Geometry check sheet. Reference: the model listing, model coordinates, mm. A direction names the side the tool comes from. Round coordinates to 2 decimals unless told otherwise and drop trailing zeros. Order: outer loops, then holes, each group sorted by start corner. A loop starts at its lowest first (then second) coordinate and runs counter-clockwise, first axis right, second up. Notation, with made-up numbers: (-1, -5.5) -> (29, -5.5) arc R8 cw to (29, -0.5) -> close; hole circle Ø7 at (-19, -28.75). An arc over 180 degrees is marked (long way). Answer as a JSON object with one key per item and string values. Group by question number.
Autodesk Inventor part; units mm, degrees
ref_plane "工作平面1" through (0, 3.5, 0) normal (0, 1, 0) x (-1, 0, 0)
ref_plane "YZ Plane" through (0, 0, 0) normal (1, 0, 0) x (0, 1, 0)
ref_plane "XY Plane" through (0, 0, 0) normal (0, 0, 1) x (1, 0, 0)
sketch "草圖1" plane through (0, 0, 0) normal (0, 1, 0) x (-1, 0, 0)
  circle A0 centre (0, 0) radius 1.75
  arc A1 (5, 0) -> (-5, 0) centre (0, 0) ccw
  circle A2 centre (0, -50) radius 1.75
  arc A3 (-5, -50) -> (5, -50) centre (0, -50) ccw
  line L0 (5, 0) -> (5, -50)
  line L1 (-5, 0) -> (-5, -50)
  dimension "d1" = 3.5
  dimension "d2" = 10
  dimension "d3" = 3.5
  dimension "d4" = 10
  dimension "d36" = 50
extrude "擠出1" add sketch "草圖1" along normal blind 7
sketch "草圖2" plane through (0, 7, 0) normal (0, 1, 0) x (1, 0, 0)
  line L0 (0, 0) -> (0, 15) construction
  line L1 (-5, 50) -> (-5, 0)
  line L2 (5, 0) -> (5, 50)
  arc A0 (-5, 0) -> (5, 0) centre (0, 0) ccw
  circle A1 centre (0, 0) radius 1.75
  line L3 (-5, 15) -> (5, 15)
  point P0 (-5, 9)
  point P1 (5, 9)
  dimension "d7" = 15
sketch "草圖3" plane through (0, 0, 0) normal (0, -1, 0) x (1, 0, 0)
  line L0 (-5, -9) -> (5, -9)
  arc A0 (5, 0) -> (-5, 0) centre (0, 0) ccw
  line L1 (-5, -50) -> (-5, 0)
  circle A1 centre (0, 0) radius 1.75
  line L2 (5, 0) -> (5, -50)
extrude "擠出2" add sketch "草圖2" along normal blind 5.5
sketch "草圖5" plane through (0, 7, 0) normal (0, 1, 0) x (1, 0, 0)
  circle A0 centre (0, 50) radius 1.75
  circle A1 centre (0, 50) radius 5
  point P0 (0, 0)
  dimension "d17" = 10
extrude "擠出5" add sketch "草圖5" along normal blind 5.5
sketch "草圖6" plane through (0, 0, 0) normal (0, -1, 0) x (1, 0, 0)
  circle A0 centre (0, -50) radius 1.75
  circle A1 centre (0, -50) radius 5
  point P0 (0, 0)
  dimension "d20" = 10
extrude "擠出6" add sketch "草圖6" along normal blind 5.5
sketch "草圖9" plane through (0, 0, 0) normal (0, -1, 0) x (1, 0, 0)
  circle A0 centre (0, 0) radius 1.75
  circle A1 centre (0, 0) radius 1.75
  line L0 (-5, -15) -> (-5, 0)
  arc A2 (5, 0) -> (-5, 0) centre (0, 0) ccw
  line L1 (5, 0) -> (5, -15)
  line L2 (5, -15) -> (-5, -15)
extrude "擠出7" add sketch "草圖9" along normal blind 5.5
sketch "草圖10" plane through (-5, 0, -50) normal (-1, 0, 0) x (0, 0, 1)
  line L0 (55, 12.5) -> (50, 12.5) construction
  line L1 (55, 12.5) -> (55, 9.5) construction
  line L2 (55, -5.5) -> (55, 12.5) construction
  line L3 (55, 9.5) -> (38, 9.5)
  line L4 (38, 9.5) -> (38, -2.5)
  line L5 (38, -2.5) -> (55, -2.5)
  line L6 (55, 9.5) -> (55, -2.5)
  point P0 (50, 0)
  dimension "d25" = 3
  dimension "d26" = 17
  dimension "d27" = 12
extrude "擠出8" cut sketch "草圖10" against normal up to next
ref_plane "工作平面1" through (0, 3.5, 0) normal (0, 1, 0) x (-1, 0, 0)
sketch "草圖11" plane through (0, 3.5, 0) normal (0, 1, 0) x (-1, 0, 0)
  circle A0 centre (0, 0) radius 1.75
  line L0 (5, -15) -> (5, 0)
  arc A1 (5, 0) -> (-5, 0) centre (0, 0) ccw
  line L1 (-5, 0) -> (-5, -15)
  line L2 (-5, -15) -> (5, -15)
  arc A2 (5, -50) -> (-5, -50) centre (0, -50) ccw
  line L3 (5, -50) -> (5, -15)
  line L4 (5, -15) -> (-5, -15)
  line L5 (-5, -15) -> (-5, -50)
  circle A3 centre (0, -50) radius 1.75
  circle A4 centre (0, -50) radius 5
  dimension "d35" = 50
properties part number "筷子套軸"
Item 1: Sectioned sample at D-D, the plane y = -4. Enter the section's corners in (x, z), then the cut area to 3 significant figures.
Item 2: Depth check by flat-ended pin: pin 1 Ø5 at (x, y) = (0.5, 0.5) entering from +Z; pin 2 Ø3 at (x, z) = (0, -50) entering from +Y; pin 3 Ø1 at (x, z) = (2, -22) entering from -Y; pin 4 Ø3 at (x, y) = (-3.5, -0.5) entering from -Z. Enter the tip coordinate at first touch or a pass-through.
Item 3: Set-up check for faces 4 (the flat face through (0, 10, -15)), 5 (the cylindrical face through (-0.651, 3.626, -54.957)), 6 (the flat face through (0, 9.5, -3)), 7 (the flat face through (5, 4, -25)): record each of +Z, -Z, +X, -X, +Y, -Y from which the full face is reachable in a straight line by a thin tool's end or side.
Item 4: Thickness scan on L1, parallel to Z at x = 0, y = 10.9; L2, parallel to X at y = 3.75, z = -50; L3, parallel to Y at x = 3.5, z = -10.5. Record the ranges inside material, lowest first.
Item 5: Sectioned sample at A-A, the plane y = -1.75. Enter the section's corners in (x, z).
Item 6: Mould release check, pull along Y, two halves, no side actions. Record for faces 1 (the flat face through (0, 4, -12)), 2 (the flat face through (0, 0, -32)), 3 (the flat face through (0, -3, -15)): pulls with the +Y half, pulls with the -Y half, needs draft (parallel to the pull), parting line crosses it, or undercut.
Item 7: Sectioned sample at B-B, the plane x = 0. Enter the section's corners in (y, z).
Item 8: Sectioned sample at C-C, the plane z = -4. Enter the section's corners in (x, y), then the cut area to 3 significant figures.
Result:
{
 "1": {"outline": "circle Ø10 at (0, -50); (-5, -15) -> (5, -15) -> (5, 0) arc R5 ccw to (-5, 0) -> close; hole circle Ø3.5 at (0, -50); hole circle Ø3.5 at (0, 0)", "area": "249 mm2"},
 "2": {"pin 1": "stops at z = -12", "pin 2": "passes through", "pin 3": "stops at y = 0", "pin 4": "stops at z = -54.58"},
 "3": {"face 4": "+X, -X, +Y", "face 5": "none", "face 6": "+Z, +X, -X", "face 7": "+Z, -Z, +X, +Y, -Y"},
 "4": {"L1": "z = -55 to -51.75, -48.25 to -45, -15 to -1.75, 1.75 to 5", "L2": "x = -5 to -1.75, 1.75 to 5", "L3": "y = -5.5 to -2.5, 9.5 to 12.5"},
 "5": {"outline": "circle Ø10 at (0, -50); (-5, -15) -> (5, -15) -> (5, -12) -> (-5, -12) -> close; hole circle Ø3.5 at (0, -50)"},
 "6": {"face 1": "undercut", "face 2": "pulls with the -Y half", "face 3": "needs draft"},
 "7": {"outline": "(-5.5, -55) -> (12.5, -55) -> (12.5, -51.75) -> (-5.5, -51.75) -> close; (-5.5, -48.25) -> (12.5, -48.25) -> (12.5, -45) -> (7, -45) -> (7, -15) -> (12.5, -15) -> (12.5, -1.75) -> (9.5, -1.75) -> (9.5, -12) -> (-2.5, -12) -> (-2.5, -1.75) -> (-5.5, -1.75) -> (-5.5, -15) -> (0, -15) -> (0, -45) -> (-5.5, -45) -> close; (-5.5, 1.75) -> (-2.5, 1.75) -> (-2.5, 5) -> (-5.5, 5) -> close; (9.5, 1.75) -> (12.5, 1.75) -> (12.5, 5) -> (9.5, 5) -> close"},
 "8": {"outline": "(-5, -5.5) -> (5, -5.5) -> (5, -2.5) -> (-5, -2.5) -> close; (-5, 9.5) -> (5, 9.5) -> (5, 12.5) -> (-5, 12.5) -> close", "area": "60.0 mm2"}
}
